from build123d import *

# Parameters (mm, degrees)
SKETCH2_R           = 9.525
BOSS_EXTRUDE1_DEPTH = 7.14375
SKETCH3_R           = 9.525
SKETCH3_R_2         = 6.746875
CUT_EXTRUDE1_DEPTH  = 2.38125
FILLET1_R           = 2.54
SKETCH4_R           = 3.96875
CUT_EXTRUDE2_DEPTH  = 20.636290542


with BuildPart() as part:
    # Sketch2 → Boss-Extrude1 (new, symmetric)
    with BuildSketch(Plane(origin=(0, 0, 0), x_dir=(1, 0, 0), z_dir=(0, 1, 0))):
        with Locations(Location((0, 0, 0), (0, 0, 270))):
            Circle(SKETCH2_R)
    extrude(amount=BOSS_EXTRUDE1_DEPTH, both=True)

    # Sketch3 → Cut-Extrude1 (cut, symmetric)
    with BuildSketch(Plane(origin=(0, 0, 0), x_dir=(1, 0, 0), z_dir=(0, 1, 0))):
        with Locations(Location((0, 0, 0), (0, 0, 270))):
            Circle(SKETCH3_R)
        with Locations(Location((0, 0, 0), (0, 0, 270))):
            Circle(SKETCH3_R_2, mode=Mode.SUBTRACT)
    extrude(amount=CUT_EXTRUDE1_DEPTH, both=True, mode=Mode.SUBTRACT)

    # Fillet1
    fillet1_edges = [part.edges().sort_by_distance(p)[0] for p in [
        (0, -7.14375, -9.525),
        (0, 7.14375, -9.525),
    ]]
    fillet(fillet1_edges, radius=FILLET1_R)

    # Sketch4 → Cut-Extrude2 (cut, through all)
    with BuildSketch(Plane(origin=(0, 7.14375, 0), x_dir=(1, 0, 0), z_dir=(0, 1, 0))):
        with Locations(Location((0, 0, 0), (0, 0, 270))):
            Circle(SKETCH4_R)
    extrude(amount=-CUT_EXTRUDE2_DEPTH, mode=Mode.SUBTRACT)


solid = part.part
Part model, mm, in its own coordinate system. A direction names the side the tool comes from. Coordinates: 2 decimals unless noted, no trailing zeros. Order: outer loops, then holes, each group sorted by start corner. A loop starts at its lowest first (then second) coordinate and runs counter-clockwise, first axis right, second up. Notation, with made-up numbers: M -38.75,67.25 L -14.75,67.25 A18 cw -14.75,92.25 Z; hole C 68,37 d7. An arc over 180 degrees is marked long. One line per question, with ' | ' between items.
Q1. Drill centre lines: line 1 (X direction, y = 1.5, z = 0); line 2 (Y direction, x = -4.5, z = -5.25); line 3 (X direction, y = -6, z = -3). Where is each one in solid material? Low to high.
A:
line 1: x = -6.75 to -3.97, 3.97 to 6.75 | line 2: y = -7.14 to -2.38, 2.38 to 7.14 | line 3: x = -8.6 to -2.6, 2.6 to 8.6
Q2. Pin check, flat tips, straight feed: P1, Ø4, axis at y = -4, z = -7, coming from the +X side; P2, Ø2, axis at x = 7.5, z = -2.5, coming from the +Y side; P3, Ø4, axis at x = 0.5, z = 0.5, coming from the -Y side; P4, Ø8, axis at y = 2, z = 7, coming from the +X side. Stop position of each tip, or through.
A:
P1: stops at x = 8.11 | P2: stops at y = 7.14 | P3: passes through | P4: stops at x = 9.03
Q3. Slice it at D-D (y = -0.5). Give the cut face in (x, z).
A:
outline: C 0,0 d13.49; hole C 0,0 d7.94
Q4. Slice it at A-A (z = 0). Give the cut face in (x, y) (3 decimals).
A:
outline: M -9.525,-4.604 A2.54 ccw -6.985,-7.144 L -3.969,-7.144 L -3.969,7.144 L -6.985,7.144 A2.54 ccw -9.525,4.604 L -9.525,2.381 L -6.747,2.381 L -6.747,-2.381 L -9.525,-2.381 Z; M 3.969,-7.144 L 6.985,-7.144 A2.54 ccw 9.525,-4.604 L 9.525,-2.381 L 6.747,-2.381 L 6.747,2.381 L 9.525,2.381 L 9.525,4.604 A2.54 ccw 6.985,7.144 L 3.969,7.144 Z
Q5. Two-plate mould, pull along Y, no slides. Class faces 3 (the face through (-3, -7.144, 3)), 4 (the face through (-6, 2.381, 4)), 5 (the face through (-3.874, 0.1, -0.86)): +Y half, -Y half, draft (parallel to the pull), parting line (faces both ways), or undercut.
A:
face 3: -Y half | face 4: undercut | face 5: draft
Q6. Slice it at B-B (x = 0). Give the cut face in (y, z) (3 decimals), and give its area (3 significant figures).
A:
outline: M -7.144,-6.985 A2.54 ccw -4.604,-9.525 L -2.381,-9.525 L -2.381,-6.747 L 2.381,-6.747 L 2.381,-9.525 L 4.604,-9.525 A2.54 ccw 7.144,-6.985 L 7.144,-3.969 L -7.144,-3.969 Z; M -7.144,3.969 L 7.144,3.969 L 7.144,6.985 A2.54 ccw 4.604,9.525 L 2.381,9.525 L 2.381,6.747 L -2.381,6.747 L -2.381,9.525 L -4.604,9.525 A2.54 ccw -7.144,6.985 Z | area: 127 mm^2
Q7. 3-axis set-ups, long thin cutter, end or side, ignore diameter. For faces 1 (the face through (4.56, -0.03, -4.97)), 2 (the face through (-5.796, 3.508, -7.559)): which of +Z, -Z, +X, -X, +Y, -Y reach the whole face in a straight line?
A:
face 1: none | face 2: +Y, -Y
